Input: part model. Units: mm. Frame: model coordinates. Face numbers are marked on the shaded views. A direction names the side the tool comes from. Give positions to 0.01 mm unless a question says otherwise; leave off trailing zeros. Loops run counter-clockwise (first coordinate to the right, second up) from the corner with the lowest first, then second, coordinate; pieces in that order, holes last. Notation, with made-up numbers: M 26.5,66.25 L 35.5,66.25 A32 ccw 35.5,104.25 Z; hole C 11,-8 d11. An arc over 180 degrees is marked long. One line per item, written item: value. Start each with the question number.
(1) Ray query, line 1 along Y through (x, z) = (25, 7.25); line 2 along Y through (x, z) = (70, 10); line 3 along Z through (x, y) = (85, 29). Return the intervals inside material, ascending. Write a range as from..to.
(2) Section D-D on z = 20.75. Output: boundary loops of the cut face in (x, y), plus the area to 3 significant figures.
(3) Section C-C on y = 30. Output: boundary loops of the cut face in (x, z).
(4) Pull-direction query (X, two-part tool) for the marked faces 1, 2, 3 and 4; classes: released by +X, released by -X, zero draft, split by the parting line, or undercut.
(5) Section A-A on z = 6. Output: boundary loops of the cut face in (x, y).
(6) Access query for the marked faces 5 and 6. Directions: +Z, -Z, +X, -X, +Y, -Y. A direction counts if a zero-diameter tool reaches every point of the face in a straight line with its end or side. Return the directions, or none.
(7) Section B-B on x = 70.5. Output: boundary loops of the cut face in (y, z), plus the area to 3 significant figures.
```python
from build123d import *

# Parameters (mm, degrees)
BOSS_EXTRUDE1_DEPTH = 30
SKETCH1_3_R         = 7
BOSS_EXTRUDE2_DEPTH = 15


with BuildPart() as part:
    # Sketch1 → Boss-Extrude1 (new body)
    with BuildSketch(Plane.XY):
        Polygon((0, 47.402622584), (100, 7), (100, 0), (0, 0), align=None)
    extrude(amount=BOSS_EXTRUDE1_DEPTH)

    # Sketch1_3 → Boss-Extrude2 (add)
    with BuildSketch(Plane.XY):
        Polygon((0, 60), (45.548089225, 60), (100, 38), (100, 7), (0, 47.402622584), align=None)
        with Locations((70, 33)):
            Circle(SKETCH1_3_R, mode=Mode.SUBTRACT)
        with Locations((25, 48)):
            Circle(SKETCH1_3_R, mode=Mode.SUBTRACT)
    extrude(amount=BOSS_EXTRUDE2_DEPTH)


solid = part.part
```
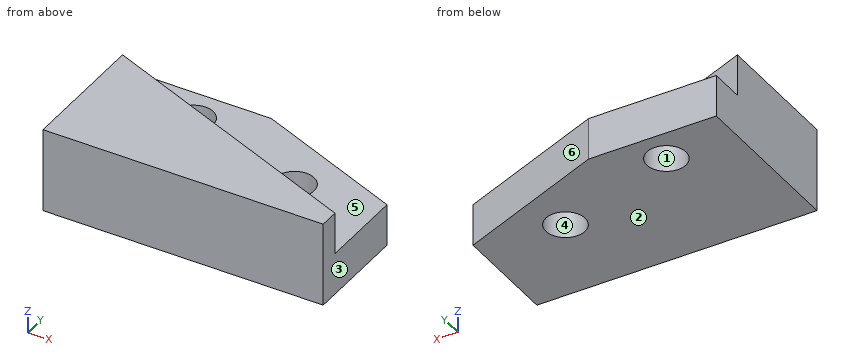
Output values:
1. line 1: y = 0..41, 55..60
1. line 2: y = 0..26, 40..50.12
1. line 3: z = 0..15
2. outline: M 0,0 L 100,0 L 100,7 L 0,47.4 Z
2. area: 2,720 mm²
3. outline: M 0,0 L 63.68,0 L 63.68,15 L 43.07,15 L 43.07,30 L 0,30 Z; M 76.32,0 L 100,0 L 100,15 L 76.32,15 Z
4. face 1: undercut
4. face 2: zero draft
4. face 3: released by +X
4. face 4: undercut
5. outline: M 0,0 L 100,0 L 100,38 L 45.55,60 L 0,60 Z; hole C 25,48 d14; hole C 70,33 d14
6. face 5: +Z, +X, +Y
6. face 6: +Z, -Z, +X, +Y
7. outline: M 0,0 L 26.02,0 L 26.02,15 L 18.92,15 L 18.92,30 L 0,30 Z; M 39.98,0 L 49.92,0 L 49.92,15 L 39.98,15 Z
7. area: 823 mm²
